Geometry check sheet. Reference: the model listing, model coordinates, mm. Face numbers are marked on the shaded views. Coordinates: 2 decimals unless noted, no trailing zeros. Loops run counter-clockwise (first coordinate to the right, second up) from the corner with the lowest first, then second, coordinate; pieces in that order, holes last. Notation, with made-up numbers: (-4, 47) - (25, 47) arc R38 cw to (25, 86) - close; hole circle Ø3 at (-14, 68). An arc over 180 degrees is marked (long way). One line per item, written item: value.
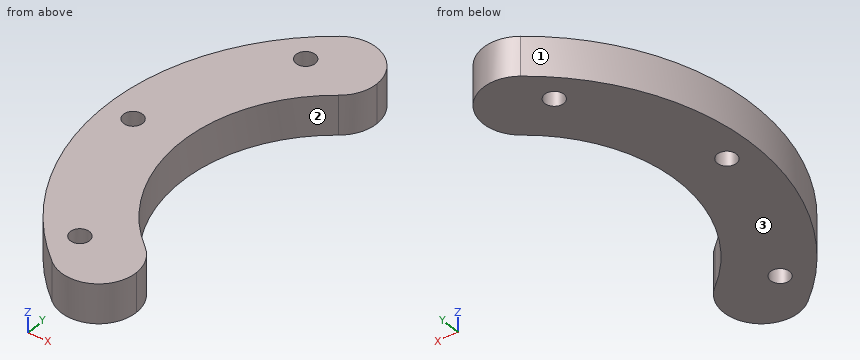
from build123d import *

# Parameters (mm, degrees)
SKETCH_1_R          = 48.25
SKETCH_1_R_2        = 32.5
SKETCH_1_R_3        = 2
EXTRUDE_1_DEPTH     = 8.3
CUT_EXTRUDE_START   = -46
SKETCH_2_R          = 2
CUT_EXTRUDE_1_DEPTH = 46


with BuildPart() as part:
    # 草图1 → 凸台-拉伸1 (new body)
    with BuildSketch(Plane.XY):
        Circle(SKETCH_1_R)
        Circle(SKETCH_1_R_2, mode=Mode.SUBTRACT)
        with Locations((0, 42.5)):
            Circle(SKETCH_1_R_3, mode=Mode.SUBTRACT)
        with Locations((30.0520382, 30.0520382)):
            Circle(SKETCH_1_R_3, mode=Mode.SUBTRACT)
        with Locations((42.5, 0)):
            Circle(SKETCH_1_R_3, mode=Mode.SUBTRACT)
        with Locations((30.0520382, -30.0520382)):
            Circle(SKETCH_1_R_3, mode=Mode.SUBTRACT)
        with Locations((0, -42.5)):
            Circle(SKETCH_1_R_3, mode=Mode.SUBTRACT)
        with Locations((-30.0520382, -30.0520382)):
            Circle(SKETCH_1_R_3, mode=Mode.SUBTRACT)
        with Locations((-42.5, 0)):
            Circle(SKETCH_1_R_3, mode=Mode.SUBTRACT)
        with Locations((-30.0520382, 30.0520382)):
            Circle(SKETCH_1_R_3, mode=Mode.SUBTRACT)
    extrude(amount=EXTRUDE_1_DEPTH)

    # 草图2 → 切除-拉伸1 (cut)
    # profile 1 of 2: a face of its own
    with BuildSketch(Plane.XY.offset(8.3).offset(CUT_EXTRUDE_START)):
        with BuildLine():
            ThreePointArc((40.5, 0), (42.5, 2), (44.5, 0))
            Line((44.5, 0), (48.25, 0))
            ThreePointArc((48.25, 0), (21.312594161, 43.287825426), (-29.421951508, 38.241486235))
            ThreePointArc((-29.421951508, 38.241486235), (-21.141442838, 39.065111353), (-16.744923335, 32))
            ThreePointArc((-16.744923335, 32), (-17.554811907, 28.521519654), (-19.817894894, 25.75851397))
            ThreePointArc((-19.817894894, 25.75851397), (14.355633318, 29.157602646), (32.5, 0))
            Line((32.5, 0), (40.5, 0))
        make_face()
        with Locations((0, 42.5)):
            Circle(SKETCH_2_R, mode=Mode.SUBTRACT)
        with Locations((30.0520382, 30.0520382)):
            Circle(SKETCH_2_R, mode=Mode.SUBTRACT)
    # profile 2 of 2: a face of its own
    with BuildSketch(Plane.XY.offset(8.3).offset(CUT_EXTRUDE_START)):
        with BuildLine():
            Line((48.25, 0), (44.5, 0))
            ThreePointArc((44.5, 0), (42.5, -2), (40.5, 0))
            Line((40.5, 0), (32.5, 0))
            ThreePointArc((32.5, 0), (14.355633349, -29.15760263), (-19.81789484, -25.758514012))
            ThreePointArc((-19.81789484, -25.758514012), (-17.554811892, -28.521519685), (-16.744923335, -32))
            ThreePointArc((-16.744923335, -32), (-21.14144309, -39.065111477), (-29.421951953, -38.241485892))
            ThreePointArc((-29.421951953, -38.241485892), (21.312593909, -43.28782555), (48.25, 0))
        make_face()
        with Locations((0, -42.5)):
            Circle(SKETCH_2_R, mode=Mode.SUBTRACT)
        with Locations((30.0520382, -30.0520382)):
            Circle(SKETCH_2_R, mode=Mode.SUBTRACT)
    extrude(amount=CUT_EXTRUDE_1_DEPTH, mode=Mode.SUBTRACT)


solid = part.part
(1) Cross-section at C-C on z = 2.5. Record the cut outline in (x, y) (3 decimals), and give its area (3 significant figures).
Reply:
outline: (-29.422, -38.241) arc R7.875 ccw to (-19.818, -25.759) arc R32.5 cw to (-19.818, 25.759) arc R7.875 ccw to (-29.422, 38.241) arc R48.25 ccw to start; hole circle Ø4 at (-42.5, 0); hole circle Ø4 at (-30.052, -30.052); hole circle Ø4 at (-30.052, 30.052)
area: 1,320 mm2
(2) Go/stop test with flat-tipped pins: pin 1 Ø4 at (x, z) = (-39, 6) entering from +Y; pin 2 Ø1.5 at (y, z) = (-30.5, 7) entering from -X; pin 3 Ø4 at (x, z) = (-33, 2.5) entering from +Y. Record where each tip stops, or that it passes through.
Reply:
pin 1: y = 30.97
pin 2: x = -37.99
pin 3: y = 36.97
(3) Cross-section at B-B on x = -18.5. Record the cut outline in (y, z), and give its area (3 significant figures).
Reply:
outline: (-36.96, 0) - (-27.04, 0) - (-27.04, 8.3) - (-36.96, 8.3) - close; (27.04, 0) - (36.96, 0) - (36.96, 8.3) - (27.04, 8.3) - close
area: 165 mm2
(4) Cross-section at D-D on x = -31. Record the cut outline in (y, z), and give its area (3 significant figures).
Reply:
outline: (-36.97, 0) - (-31.81, 0) - (-31.81, 8.3) - (-36.97, 8.3) - close; (-28.29, 0) - (-9.76, 0) - (-9.76, 8.3) - (-28.29, 8.3) - close; (9.76, 0) - (28.29, 0) - (28.29, 8.3) - (9.76, 8.3) - close; (31.81, 0) - (36.97, 0) - (36.97, 8.3) - (31.81, 8.3) - close
area: 393 mm2
(5) Material ranges on probe 1 along Y at (x, z) = (-28.5, 1); probe 2 along Y at (x, z) = (-22, 3); probe 3 along Y at (x, z) = (-21, 3.25), recorded low to high. Write a range as from..to.
Reply:
probe 1: -38.85..-31.31, -28.79..-15.62, 15.62..28.79, 31.31..38.85
probe 2: -39.43..-23.92, 23.92..39.43
probe 3: -38.99..-24.8, 24.8..38.99
(6) Cross-section at A-A on y = 0. Record the cut outline in (x, z).
Reply:
outline: (-48.25, 0) - (-44.5, 0) - (-44.5, 8.3) - (-48.25, 8.3) - close; (-40.5, 0) - (-32.5, 0) - (-32.5, 8.3) - (-40.5, 8.3) - close
(7) Release check for a two-part mould opening along Y. For the marked faces 1, 2 and 3 record: pulls with the +Y half, pulls with the -Y half, needs draft (parallel to the pull), parting line crosses it, or undercut.
Reply:
face 1: parting line crosses it
face 2: undercut
face 3: needs draft
